Geometry: final body of the model. Coordinates: model frame, mm. A direction names the side the tool comes from. Give positions to 0.01 mm unless a question says otherwise; leave off trailing zeros. Write each loop counter-clockwise with the first axis right and the second up, starting at its lowest first coordinate (ties: lowest second). Pieces come first, ordered by that corner, then holes. Notation, with made-up numbers: M 7,-9.5 L 41,-9.5 A33 ccw 41,27.5 Z; hole C 16.5,30 d9. An arc over 180 degrees is marked long. Use one line per item in the form item = value. Start each with the question number.
Item 1: Pull-direction query (Y, two-part tool) for faces 3 (the flat face through (0, 0, 0)), 4 (the conical face through (3.2, 171.7, -1)), 5 (the cylindrical face through (8.83, 163.41, -13.86)), 6 (the flat face through (-7.4, 162.687, -12.2)); classes: released by +Y, released by -Y, zero draft, split by the parting line, or undercut.
Item 2: Section query D-D on y = 160. Return loops of the section in (x, z).
Item 3: Access query for faces 1 (the flat face through (0, 172.212, 0)), 2 (the cylindrical face through (-11.016, 159.081, 8.446)). Directions: +Z, -Z, +X, -X, +Y, -Y. A direction counts if a zero-diameter tool reaches every point of the face in a straight line with its end or side. Return the directions, or none.
Item 4: Material intervals for line 1 along Y through (x, z) = (9.5, 13.5) (3 decimals); line 2 along Y through (x, z) = (-16, 2.5) (3 decimals); line 3 along Y through (x, z) = (6, 13.5) (3 decimals), sorted ascending. Write a range as from..to.
Item 5: Section query A-A on x = 0. Return loops of the section in (y, z) (3 decimals), then the cut area to 3 significant figures.
Item 6: Section query C-C on y = 116. Return loops of the section in (x, z), then the cut area to 3 significant figures.
Item 7: Contact query for flat-ended pins moving along their axis: P1, Ø10, axis at x = -7.5, y = 132.5, coming from the +Z side; P2, Ø2, axis at x = 4, y = 138, coming from the -Z side; P3, Ø10, axis at y = 36.5, z = 15, coming from the +X side. Output: stop coordinate, or through.
Item 8: Section query B-B on z = 0. Return loops of the section in (x, y) (3 decimals), then the cut area to 3 significant figures.
from build123d import *

# Parameters (mm, degrees)
SKETCH1_R           = 18.542
BOSS_EXTRUDE1_DEPTH = 155.575
SKETCH2_R           = 13.8811
BOSS_EXTRUDE2_DEPTH = 7.112
SKETCH3_R           = 16.4338
BOSS_EXTRUDE3_DEPTH = 9.525
CHAMFER1_SIZE       = 13.97
CHAMFER1_SIZE2      = 8.065583261
CHAMFER2_SIZE       = 1.524


with BuildPart() as part:
    # Sketch1 → Boss-Extrude1 (new body)
    with BuildSketch(Plane(origin=(0, 0, 0), x_dir=(1, 0, 0), z_dir=(0, 1, 0))):
        Circle(SKETCH1_R)
    extrude(amount=BOSS_EXTRUDE1_DEPTH)

    # Sketch2 → Boss-Extrude2 (add)
    with BuildSketch(Plane(origin=(0, 155.575, 0), x_dir=(1, 0, 0), z_dir=(0, 1, 0))):
        Circle(SKETCH2_R)
    extrude(amount=BOSS_EXTRUDE2_DEPTH)

    # Sketch3 → Boss-Extrude3 (add)
    with BuildSketch(Plane(origin=(0, 162.687, 0), x_dir=(1, 0, 0), z_dir=(0, 1, 0))):
        Circle(SKETCH3_R)
    extrude(amount=BOSS_EXTRUDE3_DEPTH)

    # Chamfer1
    chamfer1_edges = [part.edges().sort_by_distance(p)[0] for p in [
        (-16.4338, 172.212, 0),
    ]]
    chamfer1_side = [part.faces().sort_by_distance(p)[0] for p in [
        (0, 172.212, 0),
    ]]
    chamfer(chamfer1_edges, length=CHAMFER1_SIZE, length2=CHAMFER1_SIZE2, reference=chamfer1_side[0])

    # Chamfer2
    chamfer2_edges = [part.edges().sort_by_distance(p)[0] for p in [
        (-18.542, 0, 0),
    ]]
    chamfer(chamfer2_edges, length=CHAMFER2_SIZE)


solid = part.part
Answer sheet:
q1.face_3 = released by -Y
q1.face_4 = released by +Y
q1.face_5 = zero draft
q1.face_6 = undercut
q2.outline = C 0,0 d27.76
q3.face_1 = +Z, -Z, +X, -X, +Y
q3.face_2 = none
q4.line_1 = 0..155.575
q4.line_2 = 0..155.575, 162.687..164.285
q4.line_3 = 0..155.575, 162.687..165.105
q5.outline = M 0,-17.018 L 1.524,-18.542 L 155.575,-18.542 L 155.575,-13.881 L 162.687,-13.881 L 162.687,-16.434 L 164.146,-16.434 L 172.212,-2.464 L 172.212,2.464 L 164.146,16.434 L 162.687,16.434 L 162.687,13.881 L 155.575,13.881 L 155.575,18.542 L 1.524,18.542 L 0,17.018 Z
q5.area = 6,160 mm2
q6.outline = C 0,0 d37.08
q6.area = 1,080 mm2
q7.P1 = 18.37
q7.P2 = -18.3
q7.P3 = 15.61
q8.outline = M -18.542,1.524 L -17.018,0 L 17.018,0 L 18.542,1.524 L 18.542,155.575 L 13.881,155.575 L 13.881,162.687 L 16.434,162.687 L 16.434,164.146 L 2.464,172.212 L -2.464,172.212 L -16.434,164.146 L -16.434,162.687 L -13.881,162.687 L -13.881,155.575 L -18.542,155.575 Z
q8.area = 6,160 mm2
